CAD build for the part. Positions are in the model's coordinates, mm. Give positions to 0.01 mm unless a question says otherwise; leave off trailing zeros. Loops run counter-clockwise (first coordinate to the right, second up) from the corner with the lowest first, then second, coordinate; pieces in that order, holes last. Notation, with made-up numbers: (9, 86) -> (61, 86) arc R13 ccw to (61, 110) -> close; hole circle Ø4 at (81.25, 55). An arc over 180 degrees is marked (long way). Write each question's results on one line, items separated by ' | '. Start each with the question number.
```python
from build123d import *

# Parameters (mm, degrees)
EXTRUDE_1_DEPTH = 480
SCALE_1_SCALE   = 1.3


with BuildPart() as part:
    # 草图1 → 凸台-拉伸1 (new body)
    with BuildSketch(Plane.XY):
        with BuildLine():
            Line((-7793.3126292, 4968.547684402), (-7599.14855055, 4827.479223851))
            ThreePointArc((-7599.14855055, 4827.479223851), (-7427.939392393, 5027.939392393), (-7227.479223851, 5199.14855055))
            Line((-7227.479223851, 5199.14855055), (-7368.547684402, 5393.3126292))
            ThreePointArc((-7368.547684402, 5393.3126292), (-7531.058159836, 5261.115346452), (-7678.198873592, 5112))
            ThreePointArc((-7678.198873592, 5112), (-7737.474510483, 5041.653065761), (-7793.3126292, 4968.547684402))
        make_face()
    extrude(amount=EXTRUDE_1_DEPTH)


with BuildPart() as part_1:
    # 缩放比例1: scaled about (0, 0, 0)
    add(part.part.scale(SCALE_1_SCALE))


solid = part_1.part
```
Q1. Saw through at A-A, the plane z = 377.5. List the corners of the cut face in (x, y), then the cut area to 3 significant figures.
Q2. Saw through at B-B, the plane y = 6771. List the corners of the cut face in (x, z), then the cut area to 3 significant figures.
Q3. Saw through at C-C, the plane x = -9658.5. List the corners of the cut face in (y, z).
Q4. Drop flat-ended pins along their axis: pin 1 (6 mm diameter, centred on x = -9595, z = 373.5, fed in from -Y); pin 2 (6 mm diameter, centred on y = 6863.5, z = 464.5, fed in from -X); pin 3 (8 mm diameter, centred on y = 6409, z = 328, fed in from +X). Give the stop position or say it passes through.
Q5. Wall check: L1, parallel to Y at x = -9471.5, z = 458.5; L2, parallel to X at y = 6340, z = 520.5; L3, parallel to Y at x = -9883, z = 26. Give the ranges that are in metal, low to high.
Answer block:
1) outline: (-10131.31, 6459.11) -> (-9878.89, 6275.72) arc R2184 cw to (-9395.72, 6758.89) -> (-9579.11, 7011.31) arc R2496 ccw to start | area: 229,000 mm2
2) outline: (-9862.76, 0) -> (-9404.52, 0) -> (-9404.52, 624) -> (-9862.76, 624) -> close | area: 286,000 mm2
3) outline: (6534.14, 0) -> (6951.17, 0) -> (6951.17, 624) -> (6534.14, 624) -> close
4) pin 1: stops at y = 6592.52 | pin 2: stops at x = -9766.91 | pin 3: stops at x = -9770.5
5) L1: y = 6701.27 to 6863.19 | L2: x = -9967.36 to -9830.36 | L3: y = 6278.71 to 6750.86
